Answer from the drawing. Dimensions are ordinates in mm from the lowest x, y and z of the part. Coordinates: 2 decimals unless noted, no trailing zeros. Order: outer loops, then holes, each group sorted by start corner. A loop starts at its lowest first (then second) coordinate and runs counter-clockwise, first axis right, second up. Notation, with made-up numbers: (36.5, 87.25) - (47.5, 87.25) arc R15 cw to (47.5, 114.25) - close; hole circle Ø9 at (88, 2). An arc over 180 degrees is marked (long way). Use a Markdown table: item, result. Add a question column.
Item 1: The part is cut by section B-B, the plane x = 27.5. Give the vertices of the cut face in (y, z).
Item 2: The part is cut by section C-C, the plane y = 6. Give the vertices of the cut face in (x, z).
Item 3: The part is cut by section A-A, the plane z = 27.5. Give the vertices of the cut face in (x, y), then the cut area to 4 significant figures.
Item 4: The part is cut by section D-D, the plane y = 37.5. Give the vertices of the cut face in (x, z).
Item 5: Find the intervals of material crossed by line 1 along Y through (x, z) = (30, 52.5); line 2 along X through (y, z) = (52.5, 27); line 3 along X through (y, z) = (15, 47.5), in increasing order.
Item 6: The mould has two halves that part along Y. Classify the marked faces 1, 2, 3 and 4: released by +Y, released by -Y, zero draft, split by the parting line, or undercut.
Item 7: Flat-ended cylindrical pins translate along their axes: P1, Ø8, axis at x = 45.5, y = 33, coming from the +Z side; P2, Ø6, axis at x = 34.5, y = 38.5, coming from the +Z side; P3, Ø3, axis at y = 24.5, z = 16.5, coming from the +X side; P4, Ø6, axis at x = 43, z = 21.5, coming from the -Y side. Find the tip coordinate at first contact, or state that the pin passes through.
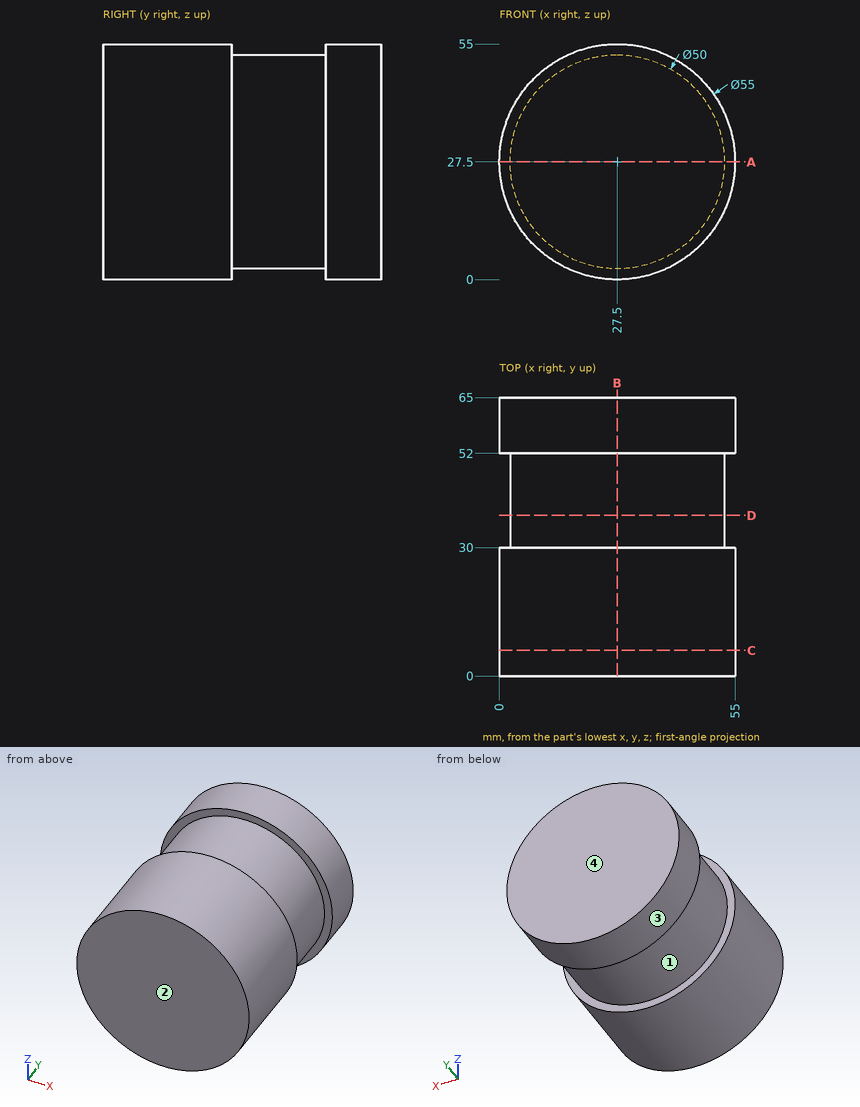
Solution:
| question | item | result |
|---|---|---|
| 1 | outline | (0, 0) - (30, 0) - (30, 2.5) - (52, 2.5) - (52, 0) - (65, 0) - (65, 55) - (52, 55) - (52, 52.5) - (30, 52.5) - (30, 55) - (0, 55) - close |
| 2 | outline | circle Ø55 at (27.5, 27.5) |
| 3 | outline | (0, 0) - (55, 0) - (55, 30) - (52.5, 30) - (52.5, 52) - (55, 52) - (55, 65) - (0, 65) - (0, 52) - (2.5, 52) - (2.5, 30) - (0, 30) - close |
| 3 | area | 3,465 mm2 |
| 4 | outline | circle Ø50 at (27.5, 27.5) |
| 5 | line 1 | y = 0 to 30, 52 to 65 |
| 5 | line 2 | x = 0 to 55 |
| 5 | line 3 | x = 8.63 to 46.37 |
| 6 | face 1 | undercut |
| 6 | face 2 | released by -Y |
| 6 | face 3 | zero draft |
| 6 | face 4 | released by +Y |
| 7 | P1 | stops at z = 50.31 |
| 7 | P2 | stops at z = 52.18 |
| 7 | P3 | stops at x = 53.31 |
| 7 | P4 | stops at y = 0 |
